CAD build for the part. Positions are in the model's coordinates, mm. Give positions to 0.01 mm unless a question says otherwise; leave off trailing zeros. Loops run counter-clockwise (first coordinate to the right, second up) from the corner with the lowest first, then second, coordinate; pieces in that order, holes last.
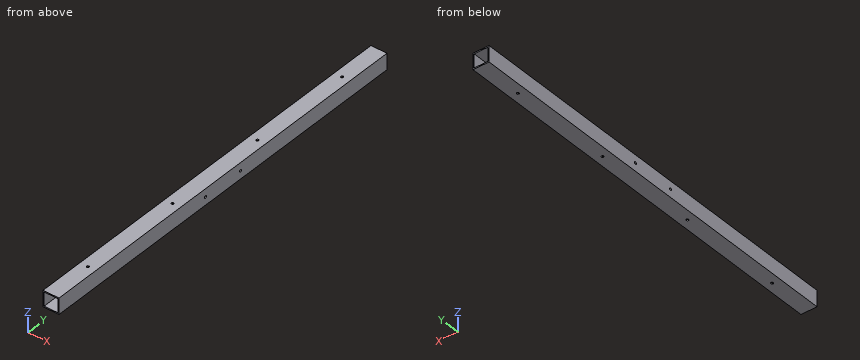
```python
from build123d import *

# Parameters (mm, degrees)
SKETCH1_W               = 44.45
SKETCH1_H               = 44.45
SKETCH1_W_2             = 38.1
SKETCH1_H_2             = 38.1
BOSS_EXTRUDE1_DEPTH     = 1130.3
F_1_4_CLEARANCE_HOLE1_D = 6.7564
F_1_4_CLEARANCE_HOLE2_D = 6.7564


with BuildPart() as part:
    # Sketch1 → Boss-Extrude1 (new body)
    with BuildSketch(Plane(origin=(0, 0, 0), x_dir=(1, 0, 0), z_dir=(0, 1, 0))):
        Rectangle(SKETCH1_W, SKETCH1_H)
        Rectangle(SKETCH1_W_2, SKETCH1_H_2, mode=Mode.SUBTRACT)
    extrude(amount=BOSS_EXTRUDE1_DEPTH)

    # 1/4 Clearance Hole1 (through all)
    with Locations(Plane.XY.offset(22.225)):
        with Locations((0, 127), (0, 1003.3), (0, 711.2), (0, 419.1)):
            Hole(F_1_4_CLEARANCE_HOLE1_D / 2)

    # 1/4 Clearance Hole2 (through all)
    with Locations(Plane(origin=(22.225, 0, 0), x_dir=(0, 0, -1), z_dir=(1, 0, 0))):
        with Locations((0, 625.475), (0, 504.825)):
            Hole(F_1_4_CLEARANCE_HOLE2_D / 2)


solid = part.part
```
1. Drop a flat-ended pin along its axis: pin 1 (6 mm diameter, centred on x = -15.5, z = -5, fed in from -Y). Give the stop position or say it passes through.
Responses:
pin 1: passes through
2. Saw through at A-A, the plane y = 732. List the corners of the cut face in (x, z) (3 decimals).
Responses:
outline: (-22.225, -22.225) - (22.225, -22.225) - (22.225, 22.225) - (-22.225, 22.225) - close; hole (-19.05, -19.05) - (19.05, -19.05) - (19.05, 19.05) - (-19.05, 19.05) - close
3. Probe line 1 along Y through (x, z) = (0, -20); line 2 along Y through (x, z) = (-21.2, 0); line 3 along X through (y, z) = (625, -16) (3 decimals). List the from-to ranges inside material, lowest first.
Responses:
line 1: y = 0 to 123.62, 130.38 to 415.72, 422.48 to 707.82, 714.58 to 999.92, 1006.68 to 1130.3
line 2: y = 0 to 501.45, 508.2 to 622.1, 628.85 to 1130.3
line 3: x = -22.225 to -19.05, 19.05 to 22.225
